Design review of the part shown in the three views and the two pictorial views. Dimensions are in mm from the part's minimum x, y and z. A direction names the side the tool comes from. Round coordinates to 2 decimals unless told otherwise and drop trailing zeros. Loops run counter-clockwise (first coordinate to the right, second up) from the corner with the lowest first, then second, coordinate; pieces in that order, holes last. Notation, with made-up numbers: (63.5, -33.5) - (101.5, -33.5) arc R26 ccw to (101.5, -5.5) - close; hole circle Ø8 at (30.25, 52). An arc over 180 degrees is marked (long way). Return JSON: item names as keys, results as strings. Group by question number.
(1) We need section B-B, the plane z = 42.5. Write out the cut boundary in (x, y), and give its area (3 significant figures).
(2) The part is to be moulded in two halves that separate along X. For the marked faces 1, 2 and 3, say which applies: pulls with the +X half, pulls with the -X half, needs draft (parallel to the pull), parting line crosses it, or undercut.
(3) Wall thickness on L1, parallel to Y at x = 28, z = 35; L2, parallel to Z at x = 40, y = 43; L3, parallel to Z at x = 92.5, y = 8.5: over which ranges is each line inside the solid? List them lowest first. Write a range as [from, to].
(4) Clearance check with flat-ended pins moving along their axes: pin 1 (20.5 mm diameter, centred on x = 101.5, y = 29, fed in from +Z); pin 2 (6 mm diameter, centred on x = 81, z = 24.5, fed in from -Y); pin 3 (5.5 mm diameter, centred on x = 26.5, z = 42, fed in from -Y). State where each tip first meets the part, or that it passes through.
(5) We need section C-C, the plane y = 49. Write out the cut boundary in (x, z), and give its area (3 significant figures).
(6) We need section A-A, the plane x = 16.5. Write out the cut boundary in (y, z).
(7) For the marked faces 4, 5, 6 and 7, list the 3-axis set-ups (+Z, -Z, +X, -X, +Y, -Y) from which the entire face can be reached by the end or side of a thin tool; tool diameter is ignored.
(8) We need section D-D, the plane z = 36. Write out the cut boundary in (x, y), and give its area (3 significant figures).
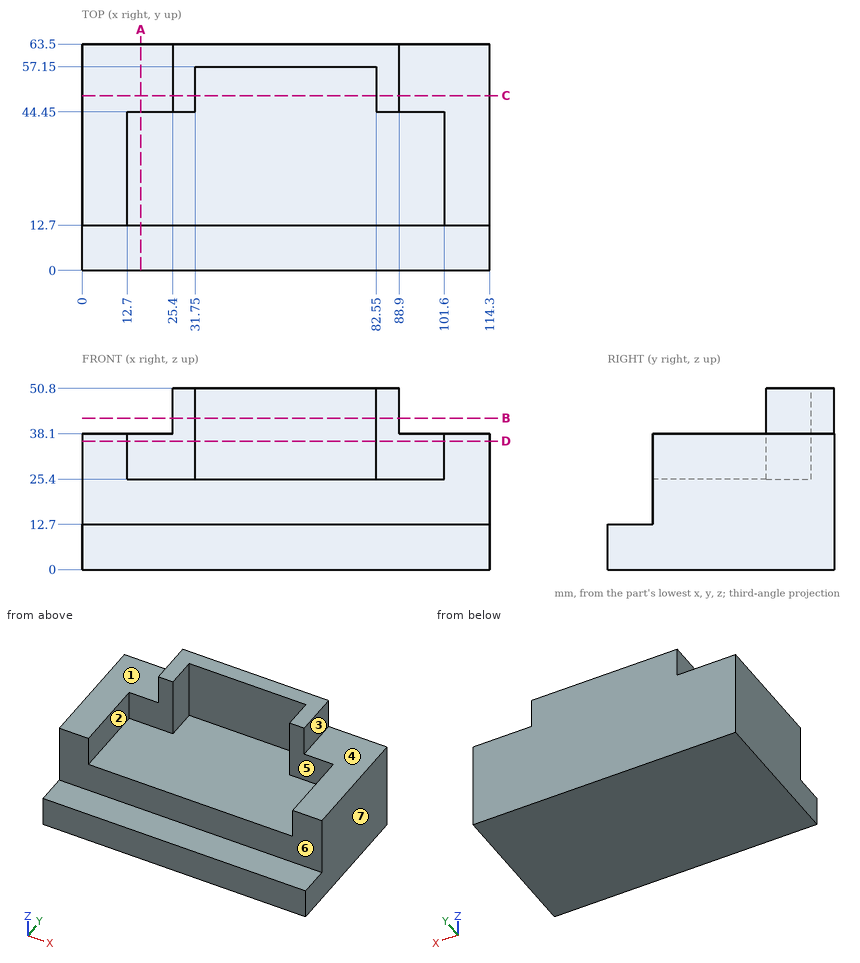
Solutions:
{
 "1": {"outline": "(25.4, 44.45) - (31.75, 44.45) - (31.75, 57.15) - (82.55, 57.15) - (82.55, 44.45) - (88.9, 44.45) - (88.9, 63.5) - (25.4, 63.5) - close", "area": "565 mm^2"},
 "2": {"face 1": "needs draft", "face 2": "undercut", "face 3": "pulls with the +X half"},
 "3": {"L1": "[44.45, 63.5]", "L2": "[0, 25.4]", "L3": "[0, 12.7]"},
 "4": {"pin 1": "z = 38.1", "pin 2": "y = 12.7", "pin 3": "y = 44.45"},
 "5": {"outline": "(0, 0) - (114.3, 0) - (114.3, 38.1) - (88.9, 38.1) - (88.9, 50.8) - (82.55, 50.8) - (82.55, 25.4) - (31.75, 25.4) - (31.75, 50.8) - (25.4, 50.8) - (25.4, 38.1) - (0, 38.1) - close", "area": "3,870 mm^2"},
 "6": {"outline": "(0, 0) - (63.5, 0) - (63.5, 38.1) - (44.45, 38.1) - (44.45, 25.4) - (12.7, 25.4) - (12.7, 12.7) - (0, 12.7) - close"},
 "7": {"face 4": "+Z, +X, +Y, -Y", "face 5": "+Z, -Y", "face 6": "+Z, +X, -X, -Y", "face 7": "+Z, -Z, +X, +Y, -Y"},
 "8": {"outline": "(0, 12.7) - (12.7, 12.7) - (12.7, 44.45) - (31.75, 44.45) - (31.75, 57.15) - (82.55, 57.15) - (82.55, 44.45) - (101.6, 44.45) - (101.6, 12.7) - (114.3, 12.7) - (114.3, 63.5) - (0, 63.5) - close", "area": "2,340 mm^2"}
}
